from build123d import *

# Parameters (mm, degrees)
SKETCH_1_W      = 95
SKETCH_1_H      = 20
SKETCH_1_W_2    = 20
SKETCH_1_W_3    = 220
EXTRUDE_4_DEPTH = 20
SKETCH_1_16_W   = 20
SKETCH_1_16_H   = 92.5
SKETCH_1_16_H_2 = 20
SKETCH_1_16_H_3 = 246.95222931
SKETCH_1_16_H_4 = 120.54777069
EXTRUDE_5_DEPTH = 20
CHAMFER_9_SIZE  = 20
CHAMFER_10_SIZE = 20


with BuildPart() as part:
    # 草图1 → 凸台-拉伸4 (new body)
    with BuildSketch(Plane(origin=(0, 0, 0), x_dir=(1, 0, 0), z_dir=(0, 1, 0))):
        with Locations((-177.5, 147.5)):
            Rectangle(SKETCH_1_W, SKETCH_1_H)
        with Locations((-120, 147.5)):
            Rectangle(SKETCH_1_W_2, SKETCH_1_H)
        with Locations((0, 147.5)):
            Rectangle(SKETCH_1_W_3, SKETCH_1_H)
        with Locations((177.5, 147.5)):
            Rectangle(SKETCH_1_W, SKETCH_1_H)
        with Locations((120, 147.5)):
            Rectangle(SKETCH_1_W_2, SKETCH_1_H)
        with Locations((177.5, -119.45222931)):
            Rectangle(SKETCH_1_W, SKETCH_1_H)
        with Locations((120, -119.45222931)):
            Rectangle(SKETCH_1_W_2, SKETCH_1_H)
        with Locations((0, -119.45222931)):
            Rectangle(SKETCH_1_W_3, SKETCH_1_H)
        with Locations((-120, -119.45222931)):
            Rectangle(SKETCH_1_W_2, SKETCH_1_H)
        with Locations((-177.5, -119.45222931)):
            Rectangle(SKETCH_1_W, SKETCH_1_H)
    extrude(amount=EXTRUDE_4_DEPTH)

    # 草图1<16> → 凸台-拉伸5 (add)
    with BuildSketch(Plane(origin=(0, 0, 0), x_dir=(1, 0, 0), z_dir=(0, 1, 0))):
        with Locations((120, 203.75)):
            Rectangle(SKETCH_1_16_W, SKETCH_1_16_H)
        with Locations((120, 147.5)):
            Rectangle(SKETCH_1_16_W, SKETCH_1_16_H_2)
        with Locations((120, 14.023885345)):
            Rectangle(SKETCH_1_16_W, SKETCH_1_16_H_3)
        with Locations((120, -119.45222931)):
            Rectangle(SKETCH_1_16_W, SKETCH_1_16_H_2)
        with Locations((120, -189.726114655)):
            Rectangle(SKETCH_1_16_W, SKETCH_1_16_H_4)
        with Locations((-120, -189.726114655)):
            Rectangle(SKETCH_1_16_W, SKETCH_1_16_H_4)
        with Locations((-120, -119.45222931)):
            Rectangle(SKETCH_1_16_W, SKETCH_1_16_H_2)
        with Locations((-120, 14.023885345)):
            Rectangle(SKETCH_1_16_W, SKETCH_1_16_H_3)
        with Locations((-120, 147.5)):
            Rectangle(SKETCH_1_16_W, SKETCH_1_16_H_2)
        with Locations((-120, 203.75)):
            Rectangle(SKETCH_1_16_W, SKETCH_1_16_H)
    extrude(amount=-EXTRUDE_5_DEPTH)

    # 倒角9
    chamfer_9_edges = [part.edges().sort_by_distance(p)[0] for p in [
        (120, 0, 129.45222931),
    ]]
    chamfer(chamfer_9_edges, length=CHAMFER_9_SIZE - 0.0001)  # a hair under: the kernel refuses the full size

    # 倒角10
    chamfer_10_edges = [part.edges().sort_by_distance(p)[0] for p in [
        (120, 0, -137.5),
        (120, 0, -157.5),
        (120, 0, 109.45222931),
        (-120, 0, 129.45222931),
        (-120, 0, 109.45222931),
        (-120, 0, -137.5),
        (-120, 0, -157.5),
    ]]
    chamfer(chamfer_10_edges, length=CHAMFER_10_SIZE - 0.0001)  # a hair under: the kernel refuses the full size


solid = part.part
Here's how the part is built. I have some questions about the finished solid (model axes, mm). A direction names the side the tool comes from. Round coordinates to 2 decimals unless told otherwise and drop trailing zeros. Order: outer loops, then holes, each group sorted by start corner. A loop starts at its lowest first (then second) coordinate and runs counter-clockwise, first axis right, second up. Notation, with made-up numbers: M 40.5,57.25 L 73.5,57.25 A22 ccw 73.5,65.25 Z; hole C 57,25 d10. An arc over 180 degrees is marked long. Return JSON: item names as keys, results as strings. Group by question number.
1. Please list where these lines run through material, in increasing order: probe 1 along X at (y, z) = (-4, 191); probe 2 along Z at (x, y) = (176, 15.5); probe 3 along Y at (x, z) = (117.5, 174.5).
2. On a 3-axis mill with a long thin cutter (end or side, diameter ignored), from which of +Z, -Z, +X, -X, +Y, -Y can I reach the whole of each face in a straight line? I mean faces 5 (the face through (-2, 0, -148)), 6 (the face through (-178, 0, -148)), 7 (the face through (-120, 0, -15)), 8 (the face through (177, 0, 119)), 9 (the face through (3, 10, 109.452)). Say none if no direction works.
3. I'm going to push flat-ended pins straight in: pin 1 Ø20 at (y, z) = (8.5, -42.5) entering from +X; pin 2 Ø16 at (x, y) = (-26, 13) entering from +Z; pin 3 Ø22 at (x, z) = (-117, 224) entering from +Y. Where does each tip first touch, or does it pass through?
4. If we section it at B-B on x = -41.5: List the corners of the cut face in (y, z) for me, then the cut area to 3 significant figures.
5. If we mould it in two halves opening along X, with no side actions, what happens to faces 1 (the face through (3, 10, -157.5)), 2 (the face through (225, 10, -147)), 3 (the face through (-119.86, 9.86, 99.31)), 4 (the face through (-2, 0, 119))? For each: pulls with the +X half, pulls with the -X half, needs draft (parallel to the pull), parting line crosses it, or undercut.
6. If we section it at A-A on y = -9: List the corners of the cut face in (x, z) for me, then the cut area to 3 significant figures.
Reply:
{
 "1": {"probe 1": "-130 to -110, 110 to 130", "probe 2": "-157.5 to -137.5, 109.45 to 129.45", "probe 3": "-20 to 0"},
 "2": {"face 5": "+Z, -Z, -Y", "face 6": "+Z, -Z, -X, -Y", "face 7": "+X, -X, +Y", "face 8": "+Z, -Z, +X, -Y", "face 9": "+Y, -Y"},
 "3": {"pin 1": "x = 130", "pin 2": "z = 129.45", "pin 3": "y = 0"},
 "4": {"outline": "M 0,-157.5 L 20,-157.5 L 20,-137.5 L 0,-137.5 Z; M 0,109.45 L 20,109.45 L 20,129.45 L 0,129.45 Z", "area": "800 mm^2"},
 "5": {"face 1": "undercut", "face 2": "pulls with the +X half", "face 3": "needs draft", "face 4": "undercut"},
 "6": {"outline": "M -130,-250 L -110,-250 L -110,250 L -130,250 Z; M 110,-250 L 130,-250 L 130,250 L 110,250 Z", "area": "20,000 mm^2"}
}
